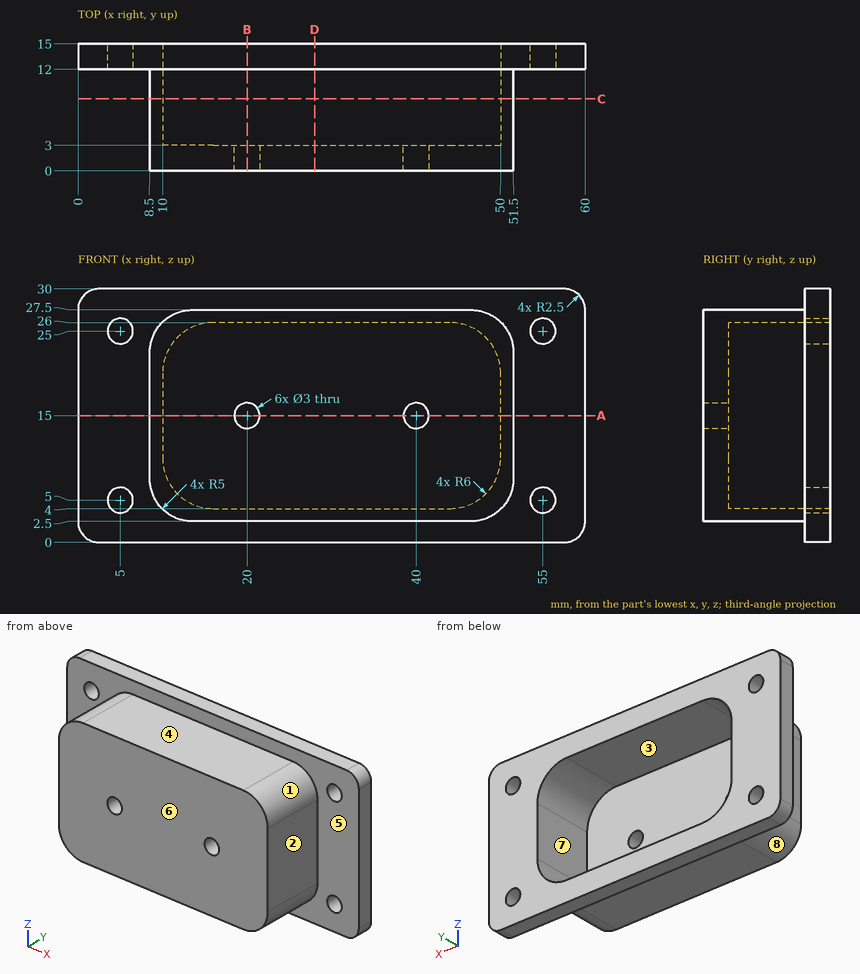
The figure shows three views and two pictorial views of one solid part (mm, origin at its lowest corner). Answer the questions. A direction names the side the tool comes from. Coordinates: 2 decimals unless noted, no trailing zeros. Loops run counter-clockwise (first coordinate to the right, second up) from the corner with the lowest first, then second, coordinate; pieces in that order, holes last. Notation, with made-up numbers: (-17.5, -20) -> (-4.5, -20) arc R16 ccw to (-4.5, 7) -> close; hole circle Ø2 at (-38, 45). An arc over 180 degrees is marked (long way). Use one line per item in the form item = value. Start each with the question number.
Item 1: The mould has two halves that part along Z. Classify the marked faces 6, 7 and 8: released by +Z, released by -Z, zero draft, split by the parting line, or undercut.
Item 2: The part is cut by section A-A on z = 15. Determine the outline of the cut face in (x, y).
Item 3: Flat-ended cylindrical pins translate along their axes: pin 1 Ø8 at (y, z) = (7.5, 14) entering from +X; pin 2 Ø8 at (x, z) = (19, 21.5) entering from +Y; pin 3 Ø6 at (y, z) = (3.5, 12.5) entering from -X; pin 4 Ø1.8 at (x, z) = (55, 5) entering from +Y. Find the tip coordinate at first contact, or state that the pin passes through.
Item 4: Consider L1, parallel to Z at x = 55, y = 13.55; L2, parallel to Z at x = 42, y = 3.5; L3, parallel to X at y = 1.5, z = 16. Determine where each line is inside the solid, lowest interval first. Write a range as [from, to].
Item 5: A tool of negligible diameter and unlimited length cuts with its end or side. For the marked faces 1, 2, 3, 4 and 5, from which of +Z, -Z, +X, -X, +Y, -Y can it reach the whole face along a straight path? Write none if from no direction.
Item 6: The part is cut by section D-D on x = 28. Determine the outline of the cut face in (y, z).
Item 7: The part is cut by section B-B on x = 20. Determine the outline of the cut face in (y, z), then the cut area to 3 significant figures.
Item 8: The part is cut by section C-C on y = 8.5. Determine the outline of the cut face in (x, z), then the cut area to 3 significant figures.
Answer key:
q1.face_6 = zero draft
q1.face_7 = undercut
q1.face_8 = released by -Z
q2.outline = (0, 12) -> (8.5, 12) -> (8.5, 0) -> (18.5, 0) -> (18.5, 3) -> (10, 3) -> (10, 15) -> (0, 15) -> close; (21.5, 0) -> (38.5, 0) -> (38.5, 3) -> (21.5, 3) -> close; (41.5, 0) -> (51.5, 0) -> (51.5, 12) -> (60, 12) -> (60, 15) -> (50, 15) -> (50, 3) -> (41.5, 3) -> close
q3.pin_1 = 51.5
q3.pin_2 = 3
q3.pin_3 = 8.5
q3.pin_4 = through
q4.L1 = [0, 3.5], [6.5, 23.5], [26.5, 30]
q4.L2 = [2.5, 4], [26, 27.5]
q4.L3 = [8.5, 18.88], [21.12, 38.88], [41.12, 51.5]
q5.face_1 = +Z, +X, -Y
q5.face_2 = +Z, -Z, +X, -Y
q5.face_3 = +Y
q5.face_4 = +Z, +X, -X, -Y
q5.face_5 = -Y
q6.outline = (0, 2.5) -> (12, 2.5) -> (12, 0) -> (15, 0) -> (15, 4) -> (3, 4) -> (3, 26) -> (15, 26) -> (15, 30) -> (12, 30) -> (12, 27.5) -> (0, 27.5) -> close
q7.outline = (0, 2.5) -> (12, 2.5) -> (12, 0) -> (15, 0) -> (15, 4) -> (3, 4) -> (3, 13.5) -> (0, 13.5) -> close; (0, 16.5) -> (3, 16.5) -> (3, 26) -> (15, 26) -> (15, 30) -> (12, 30) -> (12, 27.5) -> (0, 27.5) -> close
q7.area = 117 mm2
q8.outline = (8.5, 7.5) arc R5 ccw to (13.5, 2.5) -> (46.5, 2.5) arc R5 ccw to (51.5, 7.5) -> (51.5, 22.5) arc R5 ccw to (46.5, 27.5) -> (13.5, 27.5) arc R5 ccw to (8.5, 22.5) -> close; hole (10, 10) arc R6 ccw to (16, 4) -> (44, 4) arc R6 ccw to (50, 10) -> (50, 20) arc R6 ccw to (44, 26) -> (16, 26) arc R6 ccw to (10, 20) -> close
q8.area = 204 mm2
